Verification items for the finished model (mm, model axes). A direction names the side the tool comes from. Coordinates: 2 decimals unless noted, no trailing zeros. Loops run counter-clockwise (first coordinate to the right, second up) from the corner with the lowest first, then second, coordinate; pieces in that order, holes last.
Q1. Sectioned sample at D-D (z = -10). Enter the section's corners in (x, y).
Q2. Access from +Z, -Z, +X, -X, +Y, -Y to the whole of each face (thin tool, end or side, straight path). Record for faces 1 (the face through (20, 1, -18)), 2 (the face through (35, 1, -20.5)).
Q3. Material ranges on probe 1 along X at (y, z) = (0.35, -9); probe 2 along Z at (x, y) = (39, 0.15); probe 3 along X at (y, z) = (0.9, -17.5), recorded low to high.
Q4. Sectioned sample at C-C (z = -17.5). Enter the section's corners in (x, y), then the cut area to 3 significant figures.
Q5. Go/stop test with flat-tipped pins: P1, Ø2, axis at x = 39, z = -17.5, coming from the -Y side; P2, Ø4, axis at x = 13.3, z = -18, coming from the +Y side. Record where each tip stops, or that it passes through.
Q6. Sectioned sample at B-B (x = 4). Enter the section's corners in (y, z).
Q7. Mould release check, pull along Z, two halves, no side actions. Record for faces 3 (the face through (36.131, 0.76, -7.403)), 4 (the face through (21, 1, 0)), 5 (the face through (21, 1.5, -10)): +Z half, -Z half, draft (parallel to the pull), parting line (faces both ways), or undercut.
Q8. Sectioned sample at A-A (x = 39). Enter the section's corners in (y, z).
```python
from build123d import *

# Parameters (mm, degrees)
SKETCH_1_W          = 42
SKETCH_1_H          = 20.5
EXTRUDE_1_DEPTH     = 1.5
SKETCH_2_R          = 4
CUT_EXTRUDE_1_DEPTH = 2.5
CUT_EXTRUDE_3_REACH = 3.5
SKETCH_4_R          = 0.9
SKETCH_4_R_2        = 1.3
SKETCH_4_R_3        = 1.8
SKETCH_5_R          = 0.35
CUT_EXTRUDE_4_DEPTH = 2.5


with BuildPart() as part:
    # Эскиз1 → Бобышка-Вытянуть1 (new body)
    with BuildSketch(Plane(origin=(0, 0, 0), x_dir=(1, 0, 0), z_dir=(0, 1, 0))):
        with Locations((21, 10.25)):
            Rectangle(SKETCH_1_W, SKETCH_1_H)
    extrude(amount=EXTRUDE_1_DEPTH)

    # Эскиз2 → Вырез-Вытянуть1 (cut, through all)
    with BuildSketch(Plane(origin=(0, 1.5, 0), x_dir=(1, 0, 0), z_dir=(0, 1, 0))):
        with Locations((24, 14.5)):
            Circle(SKETCH_2_R)
        with BuildLine():
            Line((20, 20.5), (20, 14.5))
            ThreePointArc((20, 14.5), (24, 18.5), (28, 14.5))
            Line((28, 14.5), (28, 20.5))
            Line((28, 20.5), (20, 20.5))
        make_face()
    extrude(amount=-CUT_EXTRUDE_1_DEPTH, mode=Mode.SUBTRACT)

    # Эскиз4 → Вырез-Вытянуть3 (cut, up to next)
    with BuildSketch(Plane(origin=(0, 1.5, 0), x_dir=(1, 0, 0), z_dir=(0, 1, 0)), mode=Mode.PRIVATE) as cut_extrude_3_sk1:
        with BuildLine():
            Line((5.8, 20.5), (5.8, 19.8))
            ThreePointArc((5.8, 19.8), (7.3, 18.3), (8.8, 19.8))
            Line((8.8, 19.8), (8.8, 20.5))
            Line((8.8, 20.5), (5.8, 20.5))
        make_face()
    cut_extrude_3_tool1 = extrude(cut_extrude_3_sk1.sketch, amount=-CUT_EXTRUDE_3_REACH, mode=Mode.PRIVATE) & part.part
    add(cut_extrude_3_tool1.solids().sort_by_distance((7.3, 1.5, -19.531111))[0], mode=Mode.SUBTRACT)
    # Эскиз4 → Вырез-Вытянуть3 (cut, up to next)
    with BuildSketch(Plane(origin=(0, 1.5, 0), x_dir=(1, 0, 0), z_dir=(0, 1, 0)), mode=Mode.PRIVATE) as cut_extrude_3_sk2:
        with Locations((7.25, 10)):
            Circle(SKETCH_4_R)
    cut_extrude_3_tool2 = extrude(cut_extrude_3_sk2.sketch, amount=-CUT_EXTRUDE_3_REACH, mode=Mode.PRIVATE) & part.part
    add(cut_extrude_3_tool2.solids().sort_by_distance((7.25, 1.5, -10))[0], mode=Mode.SUBTRACT)
    # Эскиз4 → Вырез-Вытянуть3 (cut, up to next)
    with BuildSketch(Plane(origin=(0, 1.5, 0), x_dir=(1, 0, 0), z_dir=(0, 1, 0)), mode=Mode.PRIVATE) as cut_extrude_3_sk3:
        with Locations((30.15, 16.15)):
            Circle(SKETCH_4_R)
    cut_extrude_3_tool3 = extrude(cut_extrude_3_sk3.sketch, amount=-CUT_EXTRUDE_3_REACH, mode=Mode.PRIVATE) & part.part
    add(cut_extrude_3_tool3.solids().sort_by_distance((30.15, 1.5, -16.15))[0], mode=Mode.SUBTRACT)
    # Эскиз4 → Вырез-Вытянуть3 (cut, up to next)
    with BuildSketch(Plane(origin=(0, 1.5, 0), x_dir=(1, 0, 0), z_dir=(0, 1, 0)), mode=Mode.PRIVATE) as cut_extrude_3_sk4:
        with Locations((39, 3)):
            Circle(SKETCH_4_R_2)
    cut_extrude_3_tool4 = extrude(cut_extrude_3_sk4.sketch, amount=-CUT_EXTRUDE_3_REACH, mode=Mode.PRIVATE) & part.part
    add(cut_extrude_3_tool4.solids().sort_by_distance((39, 1.5, -3))[0], mode=Mode.SUBTRACT)
    # Эскиз4 → Вырез-Вытянуть3 (cut, up to next)
    with BuildSketch(Plane(origin=(0, 1.5, 0), x_dir=(1, 0, 0), z_dir=(0, 1, 0)), mode=Mode.PRIVATE) as cut_extrude_3_sk5:
        with Locations((39, 17.5)):
            Circle(SKETCH_4_R_2)
    cut_extrude_3_tool5 = extrude(cut_extrude_3_sk5.sketch, amount=-CUT_EXTRUDE_3_REACH, mode=Mode.PRIVATE) & part.part
    add(cut_extrude_3_tool5.solids().sort_by_distance((39, 1.5, -17.5))[0], mode=Mode.SUBTRACT)
    # Эскиз4 → Вырез-Вытянуть3 (cut, up to next)
    with BuildSketch(Plane(origin=(0, 1.5, 0), x_dir=(1, 0, 0), z_dir=(0, 1, 0)), mode=Mode.PRIVATE) as cut_extrude_3_sk6:
        with Locations((6, 3)):
            Circle(SKETCH_4_R_2)
    cut_extrude_3_tool6 = extrude(cut_extrude_3_sk6.sketch, amount=-CUT_EXTRUDE_3_REACH, mode=Mode.PRIVATE) & part.part
    add(cut_extrude_3_tool6.solids().sort_by_distance((6, 1.5, -3))[0], mode=Mode.SUBTRACT)
    # Эскиз4 → Вырез-Вытянуть3 (cut, up to next)
    with BuildSketch(Plane(origin=(0, 1.5, 0), x_dir=(1, 0, 0), z_dir=(0, 1, 0)), mode=Mode.PRIVATE) as cut_extrude_3_sk7:
        with Locations((4, 17.5)):
            Circle(SKETCH_4_R_2)
    cut_extrude_3_tool7 = extrude(cut_extrude_3_sk7.sketch, amount=-CUT_EXTRUDE_3_REACH, mode=Mode.PRIVATE) & part.part
    add(cut_extrude_3_tool7.solids().sort_by_distance((4, 1.5, -17.5))[0], mode=Mode.SUBTRACT)
    # Эскиз4 → Вырез-Вытянуть3 (cut, up to next)
    with BuildSketch(Plane(origin=(0, 1.5, 0), x_dir=(1, 0, 0), z_dir=(0, 1, 0)), mode=Mode.PRIVATE) as cut_extrude_3_sk8:
        with Locations((13.3, 18)):
            Circle(SKETCH_4_R_3)
    cut_extrude_3_tool8 = extrude(cut_extrude_3_sk8.sketch, amount=-CUT_EXTRUDE_3_REACH, mode=Mode.PRIVATE) & part.part
    add(cut_extrude_3_tool8.solids().sort_by_distance((13.3, 1.5, -18))[0], mode=Mode.SUBTRACT)
    # Эскиз4 → Вырез-Вытянуть3 (cut, up to next)
    with BuildSketch(Plane(origin=(0, 1.5, 0), x_dir=(1, 0, 0), z_dir=(0, 1, 0)), mode=Mode.PRIVATE) as cut_extrude_3_sk9:
        with Locations((35.3, 9)):
            Circle(SKETCH_4_R_3)
    cut_extrude_3_tool9 = extrude(cut_extrude_3_sk9.sketch, amount=-CUT_EXTRUDE_3_REACH, mode=Mode.PRIVATE) & part.part
    add(cut_extrude_3_tool9.solids().sort_by_distance((35.3, 1.5, -9))[0], mode=Mode.SUBTRACT)

    # Эскиз5 → Вырез-Вытянуть4 (cut, through all)
    with BuildSketch(Plane(origin=(0, 1.5, 0), x_dir=(1, 0, 0), z_dir=(0, 1, 0))):
        with Locations((29.989735949, 4.50985169)):
            Circle(SKETCH_5_R)
        with Locations((27.574921384, 3.862804077)):
            Circle(SKETCH_5_R)
        with Locations((25.932847479, 3.4228117)):
            Circle(SKETCH_5_R)
        with Locations((23.518032913, 2.775764088)):
            Circle(SKETCH_5_R)
        with Locations((30.377964517, 3.06096295)):
            Circle(SKETCH_5_R)
        with Locations((27.963149951, 2.413915338)):
            Circle(SKETCH_5_R)
        with Locations((26.321076047, 1.973922961)):
            Circle(SKETCH_5_R)
        with Locations((23.906261481, 1.326875348)):
            Circle(SKETCH_5_R)
    extrude(amount=-CUT_EXTRUDE_4_DEPTH, mode=Mode.SUBTRACT)


solid = part.part
```
Geometry check:
1. outline: (0, 0) - (6.35, 0) - (6.35, 1.5) - (0, 1.5) - close; (8.15, 0) - (33.8, 0) - (33.8, 1.5) - (8.15, 1.5) - close; (36.8, 0) - (42, 0) - (42, 1.5) - (36.8, 1.5) - close
2. face 1: -Z, +Y, -Y
2. face 2: -Z, +X, -X, +Y, -Y
3. probe 1: x = 0 to 33.5, 37.1 to 42
3. probe 2: z = -20.5 to -18.8, -16.2 to -4.3, -1.7 to 0
3. probe 3: x = 0 to 2.7, 5.3 to 11.57, 15.03 to 20, 28 to 37.7, 40.3 to 42
4. outline: (0, 0) - (2.7, 0) - (2.7, 1.5) - (0, 1.5) - close; (5.3, 0) - (11.57, 0) - (11.57, 1.5) - (5.3, 1.5) - close; (15.03, 0) - (20, 0) - (20, 1.5) - (15.03, 1.5) - close; (28, 0) - (37.7, 0) - (37.7, 1.5) - (28, 1.5) - close; (40.3, 0) - (42, 0) - (42, 1.5) - (40.3, 1.5) - close
4. area: 38.0 mm2
5. P1: passes through
5. P2: stops at y = 1.5
6. outline: (0, -20.5) - (1.5, -20.5) - (1.5, -18.8) - (0, -18.8) - close; (0, -16.2) - (1.5, -16.2) - (1.5, 0) - (0, 0) - close
7. face 3: undercut
7. face 4: +Z half
7. face 5: draft
8. outline: (0, -20.5) - (1.5, -20.5) - (1.5, -18.8) - (0, -18.8) - close; (0, -16.2) - (1.5, -16.2) - (1.5, -4.3) - (0, -4.3) - close; (0, -1.7) - (1.5, -1.7) - (1.5, 0) - (0, 0) - close
